Source: CAD feature listing. Evaluate the final solid. Frame: model axes, mm. Face numbers are marked on the shaded views. A direction names the side the tool comes from. Round coordinates to 2 decimals unless told otherwise and drop trailing zeros. Write each loop counter-clockwise with the first axis right and the second up, starting at its lowest first coordinate (ties: lowest second). Pieces come first, ordered by that corner, then holes. Notation, with made-up numbers: M 18,28.25 L 41,28.25 A12 cw 41,33.25 Z; hole C 18.5,76 d11. An arc over 180 degrees is marked long. Use a Markdown table: item, result.
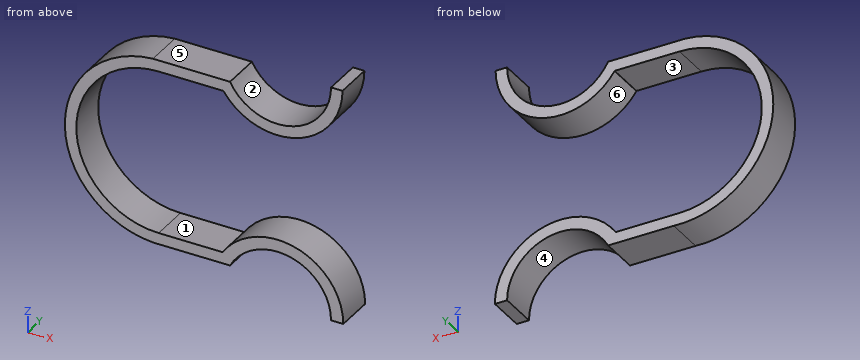
Autodesk Inventor part; units mm, degrees
ref_plane "YZ Plane" through (0, 0, 0) normal (1, 0, 0) x (0, 1, 0)
ref_plane "XZ Plane" through (0, 0, 0) normal (0, 1, 0) x (-1, 0, 0)
ref_plane "XY Plane" through (0, 0, 0) normal (0, 0, 1) x (1, 0, 0)
sketch "Sketch1" plane through (0, 0, 0) normal (0, 1, 0) x (-1, 0, 0)
  arc A0 (-7, 0) -> (7, 0) centre (0, 0) ccw
  line L0 (0, 0) -> (15.4998, -15.4998)
  line L1 (0, 0) -> (21.92, 0) construction
  arc A1 (14.3592, -26.1891) -> (7.8984, -7.8984) centre (15.4998, -15.4998) ccw
  line L2 (0, 0) -> (-7, 0)
  line L3 (15.4998, -15.4998) -> (15.4998, -4.7498)
  line L4 (15.4998, -15.4998) -> (26.2498, -15.4998) construction
  line L5 (15.4998, -4.7498) -> (5.1419, -4.7498)
  line L6 (15.4998, -15.4998) -> (15.4998, -26.2498)
  line L7 (15.4998, -15.4998) -> (37.4198, -15.4998) construction
  line L8 (15.4998, -26.2498) -> (26.0213, -26.2498) construction
  arc A2 (14.7522, -27.727) -> (16.2473, -3.2726) centre (15.4998, -15.4998) ccw
  line L9 (15.4998, -15.4998) -> (14.7522, -27.727) construction
  line L10 (15.4998, -15.4998) -> (16.2473, -3.2726) construction
  line L11 (-8.5, 0) -> (-7, 0)
  arc A3 (-8.5, 0) -> (7.0336, -4.7726) centre (0, 0) ccw
  line L12 (0, 0) -> (-8.5, 0) construction
  line L13 (0, 0) -> (8.5, 0) construction
  line L14 (7.0336, -4.7726) -> (7.0336, -3.2726)
  line L15 (7.0336, -3.2726) -> (6.1879, -3.2726)
  line L16 (7.0336, -3.2726) -> (16.2473, -3.2726)
  line L17 (14.7522, -27.727) -> (22.4821, -27.727) construction
  line L18 (15.4998, -15.4998) -> (0, -15.4998)
  line L19 (15.4998, -15.4998) -> (0, -30.9996)
  line L20 (15.4998, -15.4998) -> (37.4198, -15.4998) construction
  line L21 (14.3592, -26.1891) -> (22.4791, -26.1891) construction
  arc A4 (7, -30.9996) -> (-7, -30.9996) centre (0, -30.9996) ccw
  arc A5 (8.6, -30.9996) -> (-8.6, -30.9996) centre (0, -30.9996) ccw
  line L22 (15.4998, -26.2498) -> (7.1694, -26.2498)
  line L23 (14.7522, -27.727) -> (7.953, -27.727)
  line L24 (-8.6, -30.9996) -> (-7, -30.9996)
  line L25 (7.953, -27.727) -> (6.1879, -27.727)
  dimension "d0" = 14
  dimension "d1" = 21.92
  dimension "d2" = 45
  dimension "d3" = 21.5
  dimension "d4" = 10.75
  dimension "d5" = 90
  dimension "d6" = 90
  dimension "d13" = 12.25
  dimension "d14" = 180
  dimension "d21" = 8.5
  dimension "d22" = 180
  dimension "d23" = 1.5
  dimension "d24" = 90
  dimension "d25" = 7.0336
  dimension "d31" = 21.92
  dimension "d32" = 135
  dimension "d44" = 7
  dimension "d45" = 8.6
extrude "Extrusion3" add sketch "Sketch1" along normal blind 5 contours L5 L14 A3 L0 A0 | A0 L15 L14 L5 | L0 A3 L11 A0 | L14 L16 A2 L23 A5 L22 A1 L5 | A1 L6 L3 | A5 L25 A4 L19 | L19 A4 L24 A5
sketch "Sketch3" plane through (0, 5, 0) normal (0, 1, 0) x (1, 0, 0)
  line L0 (-15.4998, 26.2498) -> (-15.4998, 4.7498)
  arc A0 (-15.4998, 26.2498) -> (-15.4998, 4.7498) centre (-15.4998, 15.4998) ccw
  line L1 (-15.4998, 4.7498) -> (-15.4998, 15.4998)
  line L2 (-15.4998, 15.4998) -> (-15.4998, 26.2498)
  point P0 (0, 0)
extrude "Extrusion4" cut sketch "Sketch3" against normal blind 5
properties part number "small_belt_loop"
Q1. Mould query, pull axis Z, two halves, no side actions, for the marked faces 3, 4, 5 and 6. Classes: +Z half, -Z half, draft (parallel to the pull), parting line (faces both ways), or undercut.
Results are:
| item | result |
|---|---|
| face 3 | undercut |
| face 4 | -Z half |
| face 5 | +Z half |
| face 6 | undercut |
Q2. First-contact query: pin 1 Ø1 at (x, y) = (-8, 1) entering from -Z; pin 2 Ø3 at (x, z) = (3.5, -27) entering from +Y; pin 3 Ø2.5 at (x, y) = (-13, 3.5) entering from +Z. Flat tips, straight axial feed; report the tip coordinate or a pass-through.
Results are:
| item | result |
|---|---|
| pin 1 | z = -27.73 |
| pin 2 | through |
| pin 3 | z = -3.27 |
Q3. Section A-A on x = -11. Return loops of the section in (y, z), plus the area to 3 significant figures.
Results are:
| item | result |
|---|---|
| outline | M 0,-27.73 L 5,-27.73 L 5,-26.25 L 0,-26.25 Z; M 0,-4.75 L 5,-4.75 L 5,-3.27 L 0,-3.27 Z |
| area | 14.8 mm^2 |
Q4. Line query: L1, parallel to Z at x = -13, y = 1.7; L2, parallel to Z at x = -23.5, y = 1.3; L3, parallel to X at y = 4.25, z = -11. Output: solid intervals per line, ascending.
Results are:
| item | result |
|---|---|
| L1 | -27.73 to -26.25, -4.75 to -3.27 |
| L2 | -24.78 to -22.68, -8.32 to -6.22 |
| L3 | -26.89 to -25.26 |
Q5. Reachability of the marked faces 1 and 2 from +Z, -Z, +X, -X, +Y, -Y: full face, straight path, thin tool, end or side. Return the list, or none.
Results are:
| item | result |
|---|---|
| face 1 | +Y, -Y |
| face 2 | +Z, +Y, -Y |
Q6. Section B-B on z = -8. Return loops of the section in (x, y), plus the area to 3 significant figures.
Results are:
| item | result |
|---|---|
| outline | M -25.19,0 L -23.2,0 L -23.2,5 L -25.19,5 Z; M -2.87,0 L 2.87,0 L 2.87,5 L -2.87,5 Z |
| area | 38.6 mm^2 |
Q7. Section D-D on z = -14. Return loops of the section in (x, y), plus the area to 3 significant figures.
Results are:
| item | result |
|---|---|
| outline | M -27.66,0 L -26.14,0 L -26.14,5 L -27.66,5 Z |
| area | 7.57 mm^2 |
